from build123d import *

# Parameters (mm, degrees)
BOX_W             = 175
BOX_H             = 5
BOX_DEPTH         = 50
SKETCH_R          = 10
POCKET_DEPTH      = 5.001
SKETCH003_R       = 5
POCKET002_DEPTH   = 5.001
SKETCH001_R       = 18
PAD_DEPTH         = 5
SKETCH002_R       = 15
POCKET001_DEPTH   = 5.001
FUSION_ROLL_ANGLE = -90


with BuildPart() as pocket002:
    # Box → Box (new body)
    with BuildSketch(Plane.XY):
        with Locations((87.5, 2.5)):
            Rectangle(BOX_W, BOX_H)
    extrude(amount=BOX_DEPTH)

    # Sketch → Pocket (cut, through all)
    with BuildSketch(Plane.XZ):
        with Locations((31, 35)):
            Circle(SKETCH_R)
        with Locations((139, 35)):
            Circle(SKETCH_R)
    extrude(amount=-POCKET_DEPTH, mode=Mode.SUBTRACT)

    # Sketch003 → Pocket002 (cut, through all)
    with BuildSketch(Plane.XZ):
        with Locations((65, 22)):
            Circle(SKETCH003_R)
    extrude(amount=-POCKET002_DEPTH, mode=Mode.SUBTRACT)


with BuildPart() as fusion:
    # Sketch001 → Pad (new body)
    with BuildSketch(Plane.XZ):
        with Locations((65, 22)):
            Circle(SKETCH001_R)
    extrude(amount=PAD_DEPTH)

    # Sketch002 → Pocket001 (cut, through all)
    with BuildSketch(Plane.XZ.offset(5)):
        with Locations((65, 22)):
            Circle(SKETCH002_R)
    extrude(amount=-POCKET001_DEPTH, mode=Mode.SUBTRACT)

    # Fusion: union Pocket002
    add(pocket002.part)


with BuildPart() as fusion_1:
    # Fusion roll: moved
    add(fusion.part.rotate(Axis((0, 0, 0), (1, 0, 0)), FUSION_ROLL_ANGLE))


with BuildPart() as fusion_2:
    # Fusion placement: moved
    add(fusion_1.part)


solid = fusion_2.part
Verification items for the finished model (mm, model axes). A direction names the side the tool comes from. Give positions to 0.01 mm unless a question says otherwise; leave off trailing zeros. Loops run counter-clockwise (first coordinate to the right, second up) from the corner with the lowest first, then second, coordinate; pieces in that order, holes last.
1. Cross-section at C-C on z = -1.5. Record the cut outline in (x, y), and give its area (3 significant figures).
Derived:
outline: (0, 0) - (175, 0) - (175, 50) - (0, 50) - close; hole circle Ø20 at (31, 35); hole circle Ø10 at (65, 22); hole circle Ø20 at (139, 35)
area: 8,040 mm2
2. Cross-section at B-B on x = 139. Record the cut outline in (y, z), and give its area (3 significant figures).
Derived:
outline: (0, -5) - (25, -5) - (25, 0) - (0, 0) - close; (45, -5) - (50, -5) - (50, 0) - (45, 0) - close
area: 150 mm2
3. Go/stop test with flat-tipped pins: P1, Ø12, axis at x = 31, y = 35, coming from the -Z side; P2, Ø5, axis at x = 109.5, y = 23, coming from the +Z side; P3, Ø4, axis at y = 38.5, z = 3, coming from the +X side. Record where each tip stops, or that it passes through.
Derived:
P1: passes through
P2: stops at z = 0
P3: stops at x = 75.67
4. Tool access check on faces 1 (the flat face through (0, 25, -2)), 2 (the cylindrical face through (53, 13, 3)). Record the directions out of +Z, -Z, +X, -X, +Y, -Y that give a thin tool (end or side, any length) a straight path to the whole face; none if there is none.
Derived:
face 1: +Z, -Z, -X, +Y, -Y
face 2: +Z
5. Material ranges on probe 1 along Y at (x, z) = (31, -2); probe 2 along Y at (x, z) = (65, -3.25); probe 3 along X at (y, z) = (33, -3.75), recorded low to high.
Derived:
probe 1: y = 0 to 25, 45 to 50
probe 2: y = 0 to 17, 27 to 50
probe 3: x = 0 to 21.2, 40.8 to 129.2, 148.8 to 175
6. Cross-section at A-A on y = 22. Record the cut outline in (x, z).
Derived:
outline: (0, -5) - (60, -5) - (60, 0) - (50, 0) - (50, 5) - (47, 5) - (47, 0) - (0, 0) - close; (70, -5) - (175, -5) - (175, 0) - (83, 0) - (83, 5) - (80, 5) - (80, 0) - (70, 0) - close
7. Release check for a two-part mould opening along X. For faces 3 (the flat face through (61, 37, 5)), 4 (the cylindrical face through (148.237, 31.17, -2.465)), 5 (the flat face through (175, 25, -2)) record: +X half, -X half, draft (parallel to the pull), parting line (faces both ways), or undercut.
Derived:
face 3: draft
face 4: undercut
face 5: +X half
8. Cross-section at D-D on y = 35. Record the cut outline in (x, z), and give its area (3 significant figures).
Derived:
outline: (0, -5) - (21, -5) - (21, 0) - (0, 0) - close; (41, -5) - (129, -5) - (129, 0) - (77.45, 0) - (77.45, 5) - (72.48, 5) - (72.48, 0) - (57.52, 0) - (57.52, 5) - (52.55, 5) - (52.55, 0) - (41, 0) - close; (149, -5) - (175, -5) - (175, 0) - (149, 0) - close
area: 725 mm2
